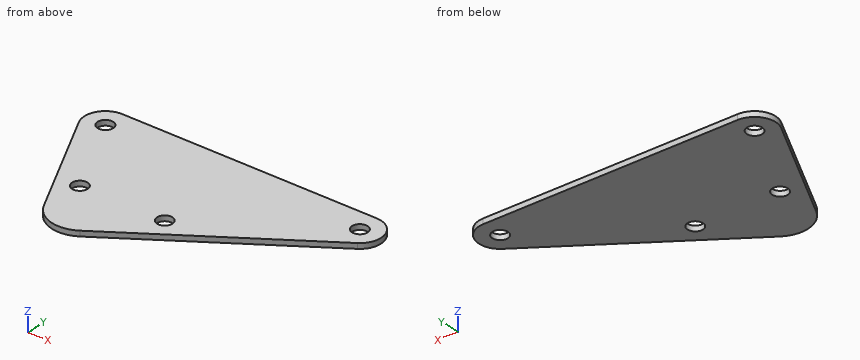
Autodesk Inventor part; units mm, degrees
ref_plane "YZ Plane" through (0, 0, 0) normal (1, 0, 0) x (0, 1, 0)
ref_plane "XZ Plane" through (0, 0, 0) normal (0, 1, 0) x (-1, 0, 0)
ref_plane "XY Plane" through (0, 0, 0) normal (0, 0, 1) x (1, 0, 0)
sketch "Sketch12" plane through (0, 0, 0) normal (0, 0, 1) x (1, 0, 0)
  circle A0 centre (0, 0) radius 2.3368
  circle A1 centre (25.4, 0) radius 2.3368
  line L0 (-10.876623, 25.4) -> (39.923377, 25.4) construction
  circle A2 centre (-12.7, 25.4) radius 2.3368
  circle A3 centre (63.5, 25.4) radius 2.3368
  circle A4 centre (63.5, 25.4) radius 6.35
  circle A5 centre (-12.7, 25.4) radius 6.35
  circle A6 centre (0, 0) radius 6.35
  circle A7 centre (25.4, 0) radius 6.35
  line L1 (-12.7, 31.75) -> (63.5, 31.75)
  line L2 (67.022346, 20.116481) -> (12.864885, -15.988494)
  line L3 (-18.379613, 22.560194) -> (-0.938054, -12.322924)
  arc A8 (-0.938054, -12.322924) -> (12.864885, -15.988494) centre (7.581365, -8.063215) ccw
  dimension "d84" = 4.6736
  dimension "d85" = 4.6736
  dimension "d86" = 25.4
  dimension "d87" = 0
  dimension "d88" = 50.8
  dimension "d89" = 25.4
  dimension "d90" = 4.6736
  dimension "d91" = 12.7
  dimension "d92" = 4.6736
  dimension "d93" = 38.1
  dimension "d94" = 12.7
  dimension "d95" = 12.7
  dimension "d96" = 12.7
  dimension "d97" = 12.7
  dimension "d98" = 9.525
extrude "Plate9" add sketch "Sketch12" along normal blind 1.5875 contours A4 | A6 | A7 | A4 L2 A8 L3 A5 L1 | A5
equation "\"d99\" = Thickness"
equation "\"BendRadius\" = Thickness"
equation "\"BendReliefWidth\" = Thickness"
equation "\"BendReliefDepth\" = 0.5 * Thickness"
equation "\"CornerReliefSize\" = 4 * Thickness"
equation "\"MinimumRemnant\" = 2 * Thickness"
equation "\"TransitionRadius\" = BendRadius"
equation "\"JacobiRadiusSize\" = BendRadius"
equation "\"GapSize\" = Thickness"
properties part number "sleds"
Could you check a few things on this model? Use its own coordinates, in mm. Round coordinates to 2 decimals unless told otherwise and drop trailing zeros. Loops run counter-clockwise (first coordinate to the right, second up) from the corner with the lowest first, then second, coordinate; pieces in that order, holes last. Notation, with made-up numbers: (-12, -13.75) - (0, -13.75) arc R20 cw to (0, 5.25) - close; hole circle Ø10 at (34, 55). An arc over 180 degrees is marked (long way). Answer in a Markdown table with one row per item. Add a question column.
(1) I need wall thicknesses on line 1 along X through (y, z) = (0.5, 0.35); line 2 along Y through (x, z) = (0, 0.6); line 3 along Y through (x, z) = (24, 0.8). Which ranges of each line are inside material? Lowest first, please.
(2) If we section it at C-C (z = 0.8): State how many separate pieces and enclosed holes the cut face has, plus the area to 3 significant figures.
(3) I'm going to push a flat-ended pin straight in: pin 1 (3.5 mm diameter, centred on x = 63.5, y = 25.4, fed in from -Z) (3 decimals). Where does the tip first touch, or does it pass through?
(4) If we section it at D-D (y = 25.4): Please give me the cut outline in (x, z).
(5) If we section it at B-B (x = 0): Please give me the cut outline in (y, z).
(6) If we section it at A-A (y = 0): Please give me the cut outline in (x, z), plus the area to 3 significant figures.
Model answer:
| question | item | result |
|---|---|---|
| 1 | line 1 | x = -7.35 to -2.28, 2.28 to 23.12, 27.68 to 37.6 |
| 1 | line 2 | y = -13.83 to -2.34, 2.34 to 31.75 |
| 1 | line 3 | y = -8.57 to -1.87, 1.87 to 31.75 |
| 2 | separate pieces | 1 |
| 2 | enclosed holes | 4 |
| 2 | area | 2,690 mm² |
| 3 | pin 1 | passes through |
| 4 | outline | (-19.05, 0) - (-15.04, 0) - (-15.04, 1.59) - (-19.05, 1.59) - close; (-10.36, 0) - (61.16, 0) - (61.16, 1.59) - (-10.36, 1.59) - close; (65.84, 0) - (69.85, 0) - (69.85, 1.59) - (65.84, 1.59) - close |
| 5 | outline | (-13.83, 0) - (-2.34, 0) - (-2.34, 1.59) - (-13.83, 1.59) - close; (2.34, 0) - (31.75, 0) - (31.75, 1.59) - (2.34, 1.59) - close |
| 6 | outline | (-7.1, 0) - (-2.34, 0) - (-2.34, 1.59) - (-7.1, 1.59) - close; (2.34, 0) - (23.06, 0) - (23.06, 1.59) - (2.34, 1.59) - close; (27.74, 0) - (36.85, 0) - (36.85, 1.59) - (27.74, 1.59) - close |
| 6 | area | 54.9 mm² |
